The listing builds one solid part. Answer for the finished solid, in the listing's coordinates (mm). Face numbers are marked on the shaded views. Round coordinates to 2 decimals unless told otherwise and drop trailing zeros. Loops run counter-clockwise (first coordinate to the right, second up) from the corner with the lowest first, then second, coordinate; pieces in that order, holes last. Notation, with made-up numbers: (59, 15) - (113, 15) arc R16 cw to (113, 45) - close; hole circle Ø1 at (18.5, 34). An arc over 180 degrees is marked (long way). Write item = value, one per line. Start each with the question number.
1) Straight lines are drawn through the part: line 1 along Y through (x, z) = (83, -1); line 2 along Y through (x, z) = (-57.5, -18.5); line 3 along Z through (x, y) = (-80, 44). For each, find the intervals that lie inside material, in ascending order.
2) Section A-A, the plane z = 5.5 is taken. Determine the outline of the cut face in (x, y), and give its area (3 significant figures).
3) For a pull along Y with two mould halves and no side action, classify the marked faces 1, 2 and 3 as released by +Y, released by -Y, zero draft, split by the parting line, or undercut.
4) Given pin 1 Ø12 at (x, y) = (11.5, 163) entering from -Z; pin 2 Ø25 at (x, z) = (32, 3.5) entering from +Y; pin 3 Ø6 at (x, y) = (-14.5, 171.5) entering from +Z, each flat-ended and moving along its own axis, determine where each tip first touches the part or whether it passes through.
5) Section B-B, the plane x = 30 is taken. Determine the outline of the cut face in (y, z), and give its area (3 significant figures).
6) Section D-D, the plane y = 180 is taken. Determine the outline of the cut face in (x, z), and give its area (3 significant figures).
7) Section C-C, the plane y = 41 is taken. Determine the outline of the cut face in (x, z), and give its area (3 significant figures).
from build123d import *

# Parameters (mm, degrees)
SKETCH22_W                   = 203.2
SKETCH22_H                   = 50.8
BASE_FLANGE2_DEPTH           = 1
EDGE_FLANGE3_STRIP_W         = 7
EDGE_FLANGE3_STRIP_H         = 1
EDGE_FLANGE3_STRIP_CUT_DEPTH = 203.2
EDGE_FLANGE3_DEPTH           = 203.2
SKETCHED_START               = -101.6
SKETCHED_BEND2_DEPTH         = 203.2
SKETCHED_BEND2_2_DEPTH       = 203.2


# Read off the part's stored shape, not the designer's step: Sketched Bend2
# Sheet-metal steps are written as plain solids
with BuildPart() as part:
    # Sketch22 → Base-Flange2 (new body)
    with BuildSketch(Plane(origin=(0, 0, 0), x_dir=(1, 0, 0), z_dir=(0, 1, 0))):
        Rectangle(SKETCH22_W, SKETCH22_H)
    extrude(amount=-BASE_FLANGE2_DEPTH)

    # Edge-Flange3 strip (across the edge) → Edge-Flange3 strip cut (cut)
    with BuildSketch(Plane(origin=(101.6, 0, -26.4), x_dir=(0, 0, 1), z_dir=(-1, 0, 0))):
        with Locations((-1.5, -0.5)):
            Rectangle(EDGE_FLANGE3_STRIP_W, EDGE_FLANGE3_STRIP_H)
    extrude(amount=EDGE_FLANGE3_STRIP_CUT_DEPTH, mode=Mode.SUBTRACT)

    # Edge-Flange3 section (across the edge) → Edge-Flange3 (add)
    with BuildSketch(Plane(origin=(101.6, 0, -26.4), x_dir=(0, 0, 1), z_dir=(-1, 0, 0))):
        with BuildLine():
            Line((0, 1), (0, 223.282))
            Line((0, 223.282), (1, 223.282))
            Line((1, 223.282), (1, 1))
            ThreePointArc((1, 1), (1.292893219, 0.292893219), (2, 0))
            Line((2, 0), (2, -1))
            ThreePointArc((2, -1), (0.585786438, -0.414213562), (0, 1))
        make_face()
    extrude(amount=EDGE_FLANGE3_DEPTH)

    # Sketched Bend2 outline → Sketched Bend2 (cut)
    with BuildSketch(Plane.YZ.offset(SKETCHED_START)):
        with BuildLine():
            ThreePointArc((153.22516494, -25.814213562), (152.576318242, -26.247759065), (151.810951377, -26.4))
            Line((151.810951377, -26.4), (223.282, -26.4))
            Line((223.282, -26.4), (223.282, -25.4))
            Line((223.282, -25.4), (153.639378502, -25.4))
            Line((153.639378502, -25.4), (153.22516494, -25.814213562))
        make_face()
    extrude(amount=SKETCHED_BEND2_DEPTH, mode=Mode.SUBTRACT)

    # Sketched Bend2 2 outline → Sketched Bend2 2 (add)
    with BuildSketch(Plane.YZ.offset(SKETCHED_START)):
        with BuildLine():
            Line((151.810951377, -25.4), (153.639378502, -25.4))
            Line((153.639378502, -25.4), (202.929787528, 23.890409026))
            Line((202.929787528, 23.890409026), (202.222680747, 24.597515807))
            Line((202.222680747, 24.597515807), (152.518058159, -25.107106781))
            ThreePointArc((152.518058159, -25.107106781), (152.19363481, -25.323879533), (151.810951377, -25.4))
        make_face()
    extrude(amount=SKETCHED_BEND2_2_DEPTH)


solid = part.part
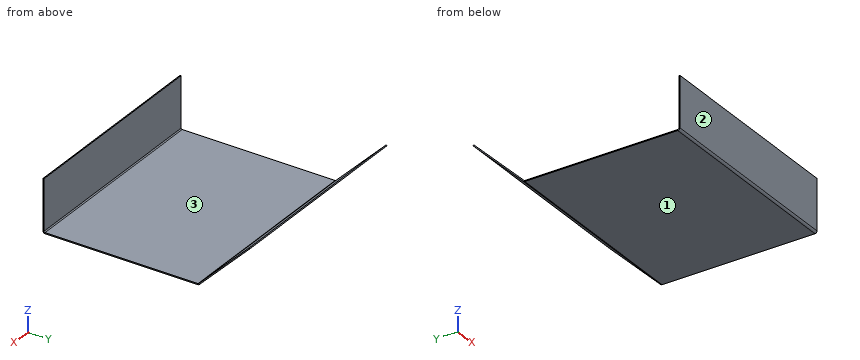
Geometry check:
q1.line_1 = -1 to 0, 176.63 to 178.04
q1.line_2 = -1 to 0, 159.13 to 160.54
q1.line_3 = -26.4 to -25.4
q2.outline = (-101.6, -1) - (101.6, -1) - (101.6, 0) - (-101.6, 0) - close; (-101.6, 183.13) - (101.6, 183.13) - (101.6, 184.54) - (-101.6, 184.54) - close
q2.area = 491 mm2
q3.face_1 = zero draft
q3.face_2 = released by -Y
q3.face_3 = undercut
q4.pin_1 = -22.04
q4.pin_2 = 195.04
q4.pin_3 = -3.13
q5.outline = (-1, -24.4) arc R2 ccw to (1, -26.4) - (151.81, -26.4) arc R2 ccw to (153.23, -25.81) - (202.93, 23.89) - (202.22, 24.6) - (152.52, -25.11) arc R1 cw to (151.81, -25.4) - (1, -25.4) arc R1 cw to (0, -24.4) - (0, 25.4) - (-1, 25.4) - close
q5.area = 274 mm2
q6.outline = (-101.6, 0.96) - (101.6, 0.96) - (101.6, 2.37) - (-101.6, 2.37) - close
q6.area = 287 mm2
q7.outline = (-101.6, -26.4) - (101.6, -26.4) - (101.6, -25.4) - (-101.6, -25.4) - close
q7.area = 203 mm2
